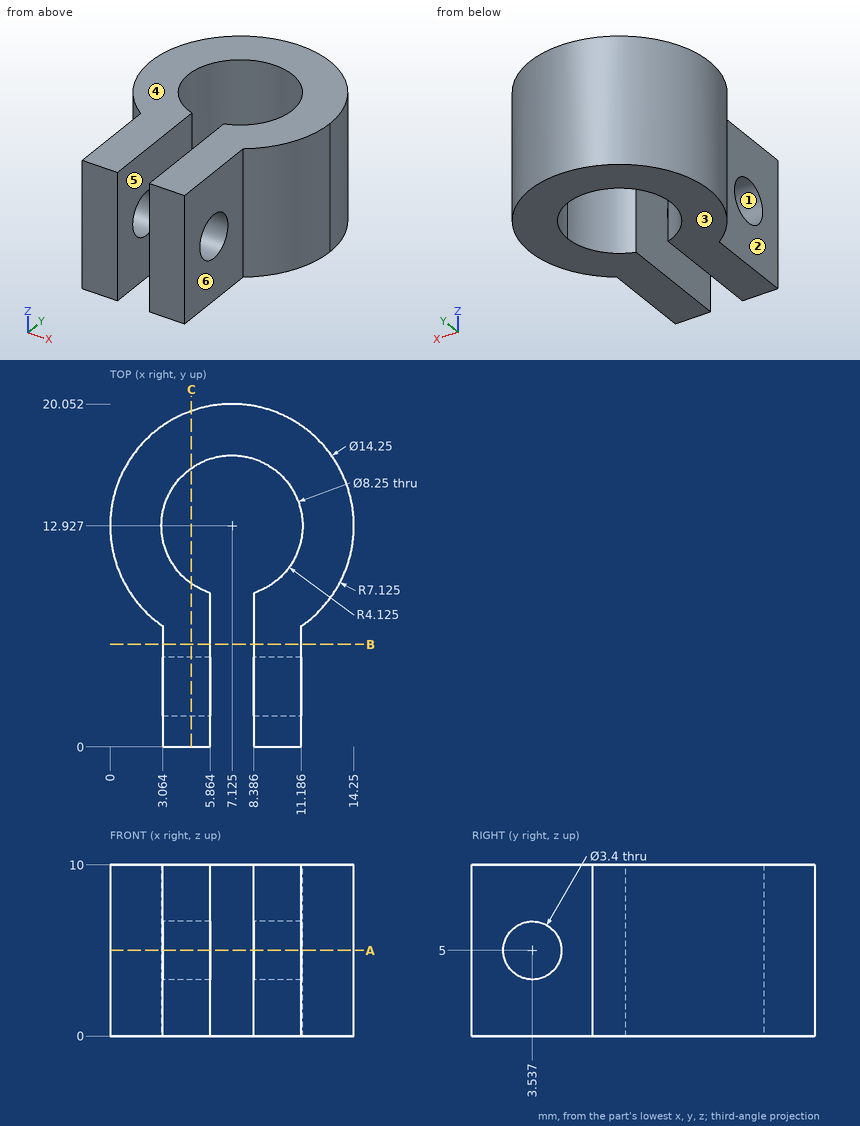
Geometry: see drawing. Coordinates: mm, zero at the bounding-box minimum. A direction names the side the tool comes from. Give positions to 0.01 mm unless a question says otherwise; leave off trailing zeros. Order: outer loops, then holes, each group sorted by start corner. A loop starts at its lowest first (then second) coordinate and runs counter-clockwise, first axis right, second up. Notation, with made-up numbers: (3.5, 13) - (30.5, 13) arc R26 ccw to (30.5, 47) - close; hole circle Ø4 at (73.5, 25). An arc over 180 degrees is marked (long way). Use a Markdown table: item, result.
(1) Access query for the marked faces 4, 5 and 6. Directions: +Z, -Z, +X, -X, +Y, -Y. A direction counts if a zero-diameter tool reaches every point of the face in a straight line with its end or side. Return the directions, or none.
Computed values:
| item | result |
|---|---|
| face 4 | +Z, +X, -X, +Y, -Y |
| face 5 | +Z, -Z, -Y |
| face 6 | +Z, -Z, +X, -Y |
(2) Section query B-B (y = 6). Output: boundary loops of the cut face in (x, z), then the cut area to 3 significant figures.
Computed values:
| item | result |
|---|---|
| outline | (3.06, 0) - (5.86, 0) - (5.86, 10) - (3.06, 10) - close; (8.39, 0) - (11.19, 0) - (11.19, 10) - (8.39, 10) - close |
| area | 56.0 mm2 |
(3) Section query A-A (z = 5). State how many separate pieces and enclosed holes the cut face has, then the cut area to 3 significant figures.
Computed values:
| item | result |
|---|---|
| separate pieces | 3 |
| enclosed holes | 0 |
| area | 115 mm2 |
(4) Draft query along Z for the marked faces 1, 2 and 3. Return one class per face: released by +Z, released by -Z, zero draft, split by the parting line, or undercut.
Computed values:
| item | result |
|---|---|
| face 1 | undercut |
| face 2 | zero draft |
| face 3 | released by -Z |
(5) Pin query (flat end, axial travel): pin 1 (2 mm diameter, centred on y = 2.5, z = 5.5, fed in from +X); pin 2 (3 mm diameter, centred on x = 11.5, z = 7.5, fed in from +Y); pin 3 (4.5 mm diameter, centred on y = 3, z = 4, fed in from -X). Return the tip coordinate at first contact, or that it passes through.
Computed values:
| item | result |
|---|---|
| pin 1 | stops at x = 11.19 |
| pin 2 | stops at y = 19.45 |
| pin 3 | stops at x = 3.06 |
(6) Line query: line 1 (X direction, y = 5, z = 8.5); line 2 (X direction, y = 9.5, z = 1.75) (1 decimal); line 3 (Y direction, x = 10.25, z = 7.25) (1 decimal). Output: solid intervals per line, ascending. Write a range as from..to.
Computed values:
| item | result |
|---|---|
| line 1 | x = 3.06..5.86, 8.39..11.19 |
| line 2 | x = 0.9..4.8, 9.4..13.4 |
| line 3 | y = 0..10.2, 15.6..19.3 |
(7) Section query C-C (x = 4.75). Output: boundary loops of the cut face in (y, z) (1 decimal).
Computed values:
| item | result |
|---|---|
| outline | (0, 0) - (9.6, 0) - (9.6, 10) - (0, 10) - close; (16.3, 0) - (19.6, 0) - (19.6, 10) - (16.3, 10) - close; hole circle Ø3.4 at (3.5, 5) |
